from build123d import *

# Parameters (mm, degrees)
F1_DEPTH = 50.8
F2_DEPTH = 1.778


with BuildPart() as f1:
    # F0 (on Front) → F1 (new body)
    with BuildSketch(Plane.XZ):
        with BuildLine():
            ThreePointArc((-75.692, 0), (-54.489303, 52.537555), (-2.759729, 75.641673))
            Line((-2.759729, 75.641673), (-2.792142, 76.530082))
            ThreePointArc((-2.792142, 76.530082), (-11.7723, 75.670751), (-20.589097, 73.761363))
            ThreePointArc((-20.589097, 73.761363), (-38.2905, 66.321091), (-53.584665, 54.711363))
            ThreePointArc((-53.584665, 54.711363), (-54.150944, 54.150944), (-54.711363, 53.584665))
            ThreePointArc((-54.711363, 53.584665), (-66.321091, 38.2905), (-73.761363, 20.589097))
            ThreePointArc((-73.761363, 20.589097), (-73.971566, 19.820621), (-74.173763, 19.05))
            ThreePointArc((-74.173763, 19.05), (-75.976807, 9.600746), (-76.581, 0))
            Line((-76.581, 0), (-75.692, 0))
        make_face()
        with BuildLine():
            ThreePointArc((2.759729, 75.641673), (52.537555, -54.489303), (-75.692, 0))
            Line((-75.692, 0), (-76.581, 0))
            ThreePointArc((-76.581, 0), (-75.976807, -9.600746), (-74.173763, -19.05))
            ThreePointArc((-74.173763, -19.05), (-73.971566, -19.820621), (-73.761363, -20.589097))
            ThreePointArc((-73.761363, -20.589097), (-66.321091, -38.2905), (-54.711363, -53.584665))
            ThreePointArc((-54.711363, -53.584665), (-54.150944, -54.150944), (-53.584665, -54.711363))
            ThreePointArc((-53.584665, -54.711363), (-38.2905, -66.321091), (-20.589097, -73.761363))
            ThreePointArc((-20.589097, -73.761363), (-19.820621, -73.971566), (-19.05, -74.173763))
            ThreePointArc((-19.05, -74.173763), (0, -76.581), (19.05, -74.173763))
            ThreePointArc((19.05, -74.173763), (19.820621, -73.971566), (20.589097, -73.761363))
            ThreePointArc((20.589097, -73.761363), (38.2905, -66.321091), (53.584665, -54.711363))
            ThreePointArc((53.584665, -54.711363), (54.150944, -54.150944), (54.711363, -53.584665))
            ThreePointArc((54.711363, -53.584665), (66.321091, -38.2905), (73.761363, -20.589097))
            ThreePointArc((73.761363, -20.589097), (73.971566, -19.820621), (74.173763, -19.05))
            ThreePointArc((74.173763, -19.05), (76.581, 0), (74.173763, 19.05))
            ThreePointArc((74.173763, 19.05), (73.971566, 19.820621), (73.761363, 20.589097))
            ThreePointArc((73.761363, 20.589097), (66.321091, 38.2905), (54.711363, 53.584665))
            ThreePointArc((54.711363, 53.584665), (54.150944, 54.150944), (53.584665, 54.711363))
            ThreePointArc((53.584665, 54.711363), (38.2905, 66.321091), (20.589097, 73.761363))
            ThreePointArc((20.589097, 73.761363), (11.7723, 75.670751), (2.792142, 76.530082))
            Line((2.792142, 76.530082), (2.759729, 75.641673))
        make_face()
    extrude(amount=-F1_DEPTH)

    # F0 (on Front) → F2 (join)
    with BuildSketch(Plane.XZ):
        with BuildLine():
            ThreePointArc((-75.692, 0), (-54.489303, 52.537555), (-2.759729, 75.641673))
            Line((-2.759729, 75.641673), (-2.792142, 76.530082))
            ThreePointArc((-2.792142, 76.530082), (-11.7723, 75.670751), (-20.589097, 73.761363))
            ThreePointArc((-20.589097, 73.761363), (-38.2905, 66.321091), (-53.584665, 54.711363))
            ThreePointArc((-53.584665, 54.711363), (-54.150944, 54.150944), (-54.711363, 53.584665))
            ThreePointArc((-54.711363, 53.584665), (-66.321091, 38.2905), (-73.761363, 20.589097))
            ThreePointArc((-73.761363, 20.589097), (-73.971566, 19.820621), (-74.173763, 19.05))
            ThreePointArc((-74.173763, 19.05), (-75.976807, 9.600746), (-76.581, 0))
            Line((-76.581, 0), (-75.692, 0))
        make_face()
        with BuildLine():
            ThreePointArc((2.759729, 75.641673), (52.537555, -54.489303), (-75.692, 0))
            Line((-75.692, 0), (-76.581, 0))
            ThreePointArc((-76.581, 0), (-75.976807, -9.600746), (-74.173763, -19.05))
            ThreePointArc((-74.173763, -19.05), (-73.971566, -19.820621), (-73.761363, -20.589097))
            ThreePointArc((-73.761363, -20.589097), (-66.321091, -38.2905), (-54.711363, -53.584665))
            ThreePointArc((-54.711363, -53.584665), (-54.150944, -54.150944), (-53.584665, -54.711363))
            ThreePointArc((-53.584665, -54.711363), (-38.2905, -66.321091), (-20.589097, -73.761363))
            ThreePointArc((-20.589097, -73.761363), (-19.820621, -73.971566), (-19.05, -74.173763))
            ThreePointArc((-19.05, -74.173763), (0, -76.581), (19.05, -74.173763))
            ThreePointArc((19.05, -74.173763), (19.820621, -73.971566), (20.589097, -73.761363))
            ThreePointArc((20.589097, -73.761363), (38.2905, -66.321091), (53.584665, -54.711363))
            ThreePointArc((53.584665, -54.711363), (54.150944, -54.150944), (54.711363, -53.584665))
            ThreePointArc((54.711363, -53.584665), (66.321091, -38.2905), (73.761363, -20.589097))
            ThreePointArc((73.761363, -20.589097), (73.971566, -19.820621), (74.173763, -19.05))
            ThreePointArc((74.173763, -19.05), (76.581, 0), (74.173763, 19.05))
            ThreePointArc((74.173763, 19.05), (73.971566, 19.820621), (73.761363, 20.589097))
            ThreePointArc((73.761363, 20.589097), (66.321091, 38.2905), (54.711363, 53.584665))
            ThreePointArc((54.711363, 53.584665), (54.150944, 54.150944), (53.584665, 54.711363))
            ThreePointArc((53.584665, 54.711363), (38.2905, 66.321091), (20.589097, 73.761363))
            ThreePointArc((20.589097, 73.761363), (11.7723, 75.670751), (2.792142, 76.530082))
            Line((2.792142, 76.530082), (2.759729, 75.641673))
        make_face()
        with BuildLine():
            Line((-139.192, 0), (-76.581, 0))
            ThreePointArc((-76.581, 0), (-75.976807, 9.600746), (-74.173763, 19.05))
            Line((-74.173763, 19.05), (-139.192, 19.05))
            Line((-139.192, 19.05), (-139.192, 0))
        make_face()
        with BuildLine():
            ThreePointArc((-74.173763, -19.05), (-75.976807, -9.600746), (-76.581, 0))
            Line((-76.581, 0), (-139.192, 0))
            Line((-139.192, 0), (-139.192, -19.05))
            Line((-139.192, -19.05), (-74.173763, -19.05))
        make_face()
        with BuildLine():
            ThreePointArc((-53.584665, 54.711363), (-38.2905, 66.321091), (-20.589097, 73.761363))
            Line((-20.589097, 73.761363), (-53.098216, 130.068808))
            Line((-53.098216, 130.068808), (-69.596, 120.543808))
            Line((-69.596, 120.543808), (-86.093784, 111.018808))
            Line((-86.093784, 111.018808), (-53.584665, 54.711363))
        make_face()
        with BuildLine():
            Line((53.098216, 130.068808), (20.589097, 73.761363))
            ThreePointArc((20.589097, 73.761363), (38.2905, 66.321091), (53.584665, 54.711363))
            Line((53.584665, 54.711363), (86.093784, 111.018808))
            Line((86.093784, 111.018808), (69.596, 120.543808))
            Line((69.596, 120.543808), (53.098216, 130.068808))
        make_face()
        with BuildLine():
            Line((-130.068808, 53.098216), (-73.761363, 20.589097))
            ThreePointArc((-73.761363, 20.589097), (-66.321091, 38.2905), (-54.711363, 53.584665))
            Line((-54.711363, 53.584665), (-111.018808, 86.093784))
            Line((-111.018808, 86.093784), (-120.543808, 69.596))
            Line((-120.543808, 69.596), (-130.068808, 53.098216))
        make_face()
        with BuildLine():
            ThreePointArc((-54.711363, -53.584665), (-66.321091, -38.2905), (-73.761363, -20.589097))
            Line((-73.761363, -20.589097), (-130.068808, -53.098216))
            Line((-130.068808, -53.098216), (-120.543808, -69.596))
            Line((-120.543808, -69.596), (-111.018808, -86.093784))
            Line((-111.018808, -86.093784), (-54.711363, -53.584665))
        make_face()
        with BuildLine():
            Line((111.018808, 86.093784), (54.711363, 53.584665))
            ThreePointArc((54.711363, 53.584665), (66.321091, 38.2905), (73.761363, 20.589097))
            Line((73.761363, 20.589097), (130.068808, 53.098216))
            Line((130.068808, 53.098216), (120.543808, 69.596))
            Line((120.543808, 69.596), (111.018808, 86.093784))
        make_face()
        with BuildLine():
            ThreePointArc((-20.589097, -73.761363), (-38.2905, -66.321091), (-53.584665, -54.711363))
            Line((-53.584665, -54.711363), (-86.093784, -111.018808))
            Line((-86.093784, -111.018808), (-69.596, -120.543808))
            Line((-69.596, -120.543808), (-53.098216, -130.068808))
            Line((-53.098216, -130.068808), (-20.589097, -73.761363))
        make_face()
        with BuildLine():
            Line((139.192, 19.05), (74.173763, 19.05))
            ThreePointArc((74.173763, 19.05), (76.581, 0), (74.173763, -19.05))
            Line((74.173763, -19.05), (139.192, -19.05))
            Line((139.192, -19.05), (139.192, 0))
            Line((139.192, 0), (139.192, 19.05))
        make_face()
        with BuildLine():
            ThreePointArc((19.05, -74.173763), (0, -76.581), (-19.05, -74.173763))
            Line((-19.05, -74.173763), (-19.05, -139.192))
            Line((-19.05, -139.192), (0, -139.192))
            Line((0, -139.192), (19.05, -139.192))
            Line((19.05, -139.192), (19.05, -74.173763))
        make_face()
        with BuildLine():
            Line((130.068808, -53.098216), (73.761363, -20.589097))
            ThreePointArc((73.761363, -20.589097), (66.321091, -38.2905), (54.711363, -53.584665))
            Line((54.711363, -53.584665), (111.018808, -86.093784))
            Line((111.018808, -86.093784), (120.543808, -69.596))
            Line((120.543808, -69.596), (130.068808, -53.098216))
        make_face()
        with BuildLine():
            ThreePointArc((53.584665, -54.711363), (38.2905, -66.321091), (20.589097, -73.761363))
            Line((20.589097, -73.761363), (53.098216, -130.068808))
            Line((53.098216, -130.068808), (69.596, -120.543808))
            Line((69.596, -120.543808), (86.093784, -111.018808))
            Line((86.093784, -111.018808), (53.584665, -54.711363))
        make_face()
    extrude(amount=-F2_DEPTH)


solid = f1.part
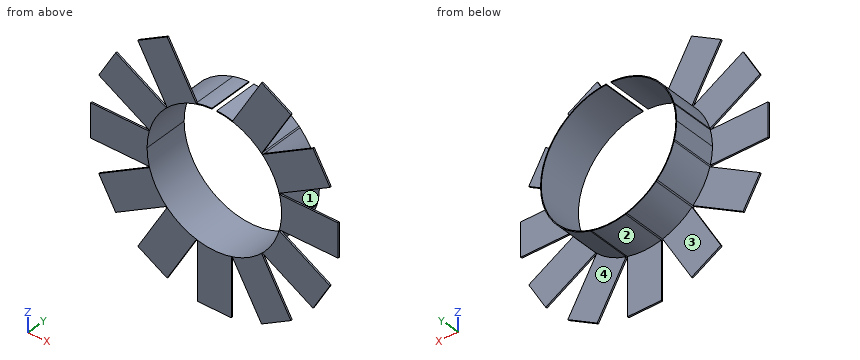
For this review, take the finished solid that the model builds, in its own axes (mm). Face numbers are marked on the shaded views. A direction names the side the tool comes from. Round coordinates to 2 decimals unless told otherwise and drop trailing zeros. Loops run counter-clockwise (first coordinate to the right, second up) from the corner with the lowest first, then second, coordinate; pieces in that order, holes last. Notation, with made-up numbers: (55.25, 64) - (86.25, 64) arc R25 cw to (86.25, 78) - close; hole circle Ø9 at (-31.75, 81.5). An arc over 180 degrees is marked (long way). Use one line per item in the form item = value.
Item 1: For line 1 (X direction, y = 37, z = -3); line 2 (X direction, y = 17.5, z = 0); line 3 (Y direction, x = -95.5, z = 45.5), list the stretches that pass through material, from the lowest coordinate up.
Answers:
line_1 = -76.52 to -75.63, 75.63 to 76.52
line_2 = -76.58 to -75.69, 75.69 to 76.58
line_3 = 0 to 1.78
Item 2: Consider section B-B on y = 44. Write out the cut boundary in (x, z), then the cut area to 3 significant figures.
Answers:
outline = (-76.58, 0) arc R76.58 ccw to (-74.17, -19.05) arc R76.58 ccw to (-73.76, -20.59) arc R76.58 ccw to (-54.71, -53.58) arc R76.59 ccw to (-53.58, -54.71) arc R76.58 ccw to (-20.59, -73.76) arc R76.58 ccw to (-19.05, -74.17) arc R76.58 ccw to (19.05, -74.17) arc R76.58 ccw to (20.59, -73.76) arc R76.58 ccw to (53.58, -54.71) arc R76.59 ccw to (54.71, -53.58) arc R76.58 ccw to (73.76, -20.59) arc R76.58 ccw to (74.17, -19.05) arc R76.58 ccw to (74.17, 19.05) arc R76.58 ccw to (73.76, 20.59) arc R76.58 ccw to (54.71, 53.58) arc R76.59 ccw to (53.58, 54.71) arc R76.58 ccw to (20.59, 73.76) arc R76.58 ccw to (2.79, 76.53) - (2.76, 75.64) arc R75.69 cw (long way) to (-2.76, 75.64) - (-2.79, 76.53) arc R76.58 ccw to (-20.59, 73.76) arc R76.58 ccw to (-53.58, 54.71) arc R76.59 ccw to (-54.71, 53.58) arc R76.58 ccw to (-73.76, 20.59) arc R76.58 ccw to (-74.17, 19.05) arc R76.58 ccw to start
area = 420 mm^2
Item 3: Clearance check with flat-ended pins moving along their axes: P1, Ø12, axis at y = 23, z = -44.5, coming from the -X side; P2, Ø12, axis at x = 68, z = 58.5, coming from the -Y side; P3, Ø19.5, axis at x = -69, z = -103.5, coming from the +Y side; P4, Ø0.9, axis at y = 0.5, z = -118, coming from the -X side. State where each tip first meets the part, or that it passes through.
Answers:
P1 = -66.2
P2 = 0
P3 = 1.78
P4 = -74.78
Item 4: Tool access review of the marked faces 1, 2, 3 and 4: name each direction out of +Z, -Z, +X, -X, +Y, -Y from which nothing blocks a thin tool from reaching the whole face with its end or side.
Answers:
face_1 = +X, +Y
face_2 = -Z, +Y
face_3 = -Z, -X, +Y
face_4 = -Z, +X, +Y
Item 5: Consider section A-A on z = -8.5. Write out the cut boundary in (x, y), then the cut area to 3 significant figures.
Answers:
outline = (-139.19, 0) - (-75.21, 0) - (-75.21, 50.8) - (-76.11, 50.8) - (-76.11, 1.78) - (-139.19, 1.78) - close; (75.21, 0) - (139.19, 0) - (139.19, 1.78) - (76.11, 1.78) - (76.11, 50.8) - (75.21, 50.8) - close
area = 315 mm^2
Item 6: Consider section D-D on z = -123. Write out the cut boundary in (x, y), then the cut area to 3 significant figures.
Answers:
outline = (-65.34, 0) - (-49.02, 0) - (-49.02, 1.78) - (-65.34, 1.78) - close; (-19.05, 0) - (19.05, 0) - (19.05, 1.78) - (-19.05, 1.78) - close; (49.02, 0) - (65.34, 0) - (65.34, 1.78) - (49.02, 1.78) - close
area = 126 mm^2
Item 7: Consider section C-C on x = 101. Write out the cut boundary in (y, z), then the cut area to 3 significant figures.
Answers:
outline = (0, -80.31) - (1.78, -80.31) - (1.78, -36.32) - (0, -36.32) - close; (0, -19.05) - (1.78, -19.05) - (1.78, 19.05) - (0, 19.05) - close; (0, 36.32) - (1.78, 36.32) - (1.78, 80.31) - (0, 80.31) - close
area = 224 mm^2
